Can you work these out from the model? Positions are in its coordinate system, mm. A direction names the side the tool comes from. Coordinates: 2 decimals unless noted, no trailing zeros. Write each loop counter-clockwise with the first axis right and the second up, starting at its lowest first coordinate (ties: lowest second). Pieces come first, ordered by that corner, then holes. Notation, with made-up numbers: M 15.5,-36.5 L 67.5,-36.5 A27 ccw 67.5,-8.5 Z; hole C 46.5,-16 d1. An arc over 180 degrees is marked long. Answer as a JSON object with one key per item and string values. Group by question number.
from build123d import *

# Parameters (mm, degrees)
SKETCH_1_W      = 41
SKETCH_1_H      = 41
EXTRUDE_1_DEPTH = 4
SKETCH_2_R      = 10
EXTRUDE_2_DEPTH = 2
SKETCH_3_R      = 2.5
EXTRUDE_3_DEPTH = 10.5


with BuildPart() as part:
    # 草图1 → 凸台-拉伸1 (new body)
    with BuildSketch(Plane(origin=(0, 0, 0), x_dir=(1, 0, 0), z_dir=(0, 1, 0))):
        Rectangle(SKETCH_1_W, SKETCH_1_H)
    extrude(amount=EXTRUDE_1_DEPTH)

    # 草图2 → 凸台-拉伸2 (add)
    with BuildSketch(Plane(origin=(0, 4, 0), x_dir=(1, 0, 0), z_dir=(0, 1, 0))):
        with Locations(Location((0, 0, 0), (0, 0, 270))):
            Circle(SKETCH_2_R)
    extrude(amount=EXTRUDE_2_DEPTH)

    # 草图3 → 凸台-拉伸3 (add)
    with BuildSketch(Plane(origin=(0, 6, 0), x_dir=(1, 0, 0), z_dir=(0, 1, 0))):
        with Locations(Location((0, 0, 0), (0, 0, 90))):
            Circle(SKETCH_3_R)
    extrude(amount=EXTRUDE_3_DEPTH)


solid = part.part
Q1. If we section it at A-A on x = 0: List the corners of the cut face in (y, z) for me, and give its area (4 significant figures).
Q2. Please list where these lines run through material, in increasing order: L1, parallel to Y at x = 12, z = -12; L2, parallel to X at y = 8.75, z = 0; L3, parallel to Y at x = -5, z = -4.
Q3. Will this pin go through, and if not, where does the flat tip stop? pin 1 (1.5 mm diameter, centred on x = 1.5, y = 12.5, fed in from -Z).
Q4. If we section it at C-C on y = 5.25: List the corners of the cut face in (x, z) for me.
Q5. On a 3-axis mill with a long thin cutter (end or side, diameter ignored), from which of +Z, -Z, +X, -X, +Y, -Y can I reach the whole of each face in a straight line? I mean faces 1 (the cylindrical face through (2.44, 11.18, 0.54)), 2 (the flat face through (0, 16.5, 0)). Say none if no direction works.
Q6. If we section it at D-D on x = -9: List the corners of the cut face in (y, z) for me, and give its area (3 significant figures).
Q7. If we section it at B-B on z = 0: List the corners of the cut face in (x, y) for me, and give its area (4 significant figures).
Reply:
{
 "1": {"outline": "M 0,-20.5 L 4,-20.5 L 4,-10 L 6,-10 L 6,-2.5 L 16.5,-2.5 L 16.5,2.5 L 6,2.5 L 6,10 L 4,10 L 4,20.5 L 0,20.5 Z", "area": "256.5 mm^2"},
 "2": {"L1": "0 to 4", "L2": "-2.5 to 2.5", "L3": "0 to 6"},
 "3": {"pin 1": "z = -2.38"},
 "4": {"outline": "C 0,0 d20"},
 "5": {"face 1": "+Y", "face 2": "+Z, -Z, +X, -X, +Y"},
 "6": {"outline": "M 0,-20.5 L 4,-20.5 L 4,-4.36 L 6,-4.36 L 6,4.36 L 4,4.36 L 4,20.5 L 0,20.5 Z", "area": "181 mm^2"},
 "7": {"outline": "M -20.5,0 L 20.5,0 L 20.5,4 L 10,4 L 10,6 L 2.5,6 L 2.5,16.5 L -2.5,16.5 L -2.5,6 L -10,6 L -10,4 L -20.5,4 Z", "area": "256.5 mm^2"}
}
